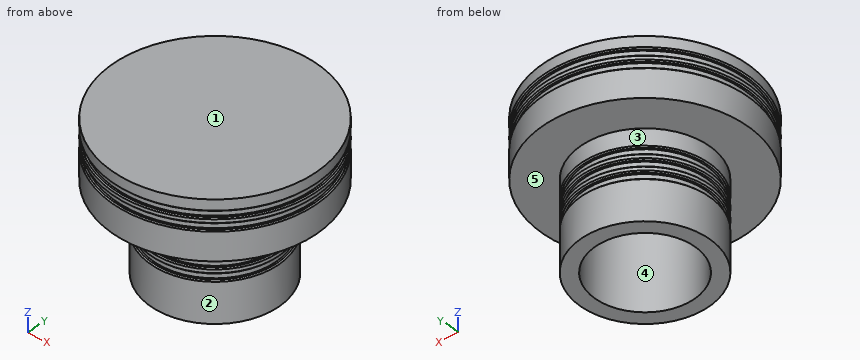
from build123d import *

# Parameters (mm, degrees)
F0_R      = 11
F0_R_2    = 8.5
F1_DEPTH  = 15
F2_R      = 17.5
F3_DEPTH  = 10
F4_R      = 11
F4_R_2    = 10.5
F5_DEPTH  = 12
F6_R      = 11
F6_R_2    = 10.5
F7_DEPTH  = 11
F8_R      = 11
F8_R_2    = 10.5
F9_DEPTH  = 10
F10_R     = 11
F10_R_2   = 10.5
F11_DEPTH = 9
F12_R     = 11
F12_R_2   = 10.5
F13_DEPTH = 8
F14_R     = 11
F14_R_2   = 10.5
F15_DEPTH = 7
F16_R     = 17.5
F16_R_2   = 17
F17_DEPTH = 8
F18_R     = 17.5
F18_R_2   = 17
F19_DEPTH = 7
F20_R     = 17.5
F20_R_2   = 17
F21_DEPTH = 6
F22_R     = 17.5
F22_R_2   = 17
F23_DEPTH = 5
F24_SIZE  = 0.2


with BuildPart() as f1:
    # F0 (on Top) → F1 (new body)
    with BuildSketch(Plane.XY):
        Circle(F0_R)
        Circle(F0_R_2, mode=Mode.SUBTRACT)
    extrude(amount=F1_DEPTH)

    # F2 (on face) → F3 (join)
    with BuildSketch(Plane.XY.offset(15)):
        Circle(F2_R)
    extrude(amount=F3_DEPTH)

    # F4 (on face) → F5 (cut)
    with BuildSketch(Plane(origin=(0, 0, 0), x_dir=(1, 0, 0), z_dir=(0, 0, -1))):
        Circle(F4_R)
        Circle(F4_R_2, mode=Mode.SUBTRACT)
    extrude(amount=-F5_DEPTH, mode=Mode.SUBTRACT)

    # F6 (on face) → F7 (join)
    with BuildSketch(Plane(origin=(0, 0, 0), x_dir=(1, 0, 0), z_dir=(0, 0, -1))):
        Circle(F6_R)
        Circle(F6_R_2, mode=Mode.SUBTRACT)
    extrude(amount=-F7_DEPTH)

    # F8 (on face) → F9 (cut)
    with BuildSketch(Plane(origin=(0, 0, 0), x_dir=(1, 0, 0), z_dir=(0, 0, -1))):
        Circle(F8_R)
        Circle(F8_R_2, mode=Mode.SUBTRACT)
    extrude(amount=-F9_DEPTH, mode=Mode.SUBTRACT)

    # F10 (on face) → F11 (join)
    with BuildSketch(Plane(origin=(0, 0, 0), x_dir=(1, 0, 0), z_dir=(0, 0, -1))):
        Circle(F10_R)
        Circle(F10_R_2, mode=Mode.SUBTRACT)
    extrude(amount=-F11_DEPTH)

    # F12 (on face) → F13 (cut)
    with BuildSketch(Plane(origin=(0, 0, 0), x_dir=(1, 0, 0), z_dir=(0, 0, -1))):
        Circle(F12_R)
        Circle(F12_R_2, mode=Mode.SUBTRACT)
    extrude(amount=-F13_DEPTH, mode=Mode.SUBTRACT)

    # F14 (on face) → F15 (join)
    with BuildSketch(Plane(origin=(0, 0, 0), x_dir=(1, 0, 0), z_dir=(0, 0, -1))):
        Circle(F14_R)
        Circle(F14_R_2, mode=Mode.SUBTRACT)
    extrude(amount=-F15_DEPTH)

    # F16 (on face) → F17 (cut)
    with BuildSketch(Plane(origin=(0, 0, 15), x_dir=(1, 0, 0), z_dir=(0, 0, -1))):
        Circle(F16_R)
        Circle(F16_R_2, mode=Mode.SUBTRACT)
    extrude(amount=-F17_DEPTH, mode=Mode.SUBTRACT)

    # F18 (on face) → F19 (join)
    with BuildSketch(Plane(origin=(0, 0, 15), x_dir=(1, 0, 0), z_dir=(0, 0, -1))):
        Circle(F18_R)
        Circle(F18_R_2, mode=Mode.SUBTRACT)
    extrude(amount=-F19_DEPTH)

    # F20 (on face) → F21 (cut)
    with BuildSketch(Plane(origin=(0, 0, 15), x_dir=(1, 0, 0), z_dir=(0, 0, -1))):
        Circle(F20_R)
        Circle(F20_R_2, mode=Mode.SUBTRACT)
    extrude(amount=-F21_DEPTH, mode=Mode.SUBTRACT)

    # F22 (on face) → F23 (join)
    with BuildSketch(Plane(origin=(0, 0, 15), x_dir=(1, 0, 0), z_dir=(0, 0, -1))):
        Circle(F22_R)
        Circle(F22_R_2, mode=Mode.SUBTRACT)
    extrude(amount=-F23_DEPTH)

    # F24
    f24_edges = [f1.edges().sort_by_distance(p)[0] for p in [
        (-17.5, 0, 23),
        (-17.5, 0, 22),
        (-17.5, 0, 20),
        (-17.5, 0, 21),
        (-11, 0, 12),
        (-11, 0, 10),
        (-11, 0, 11),
        (-11, 0, 9),
        (-11, 0, 8),
        (-11, 0, 7),
    ]]
    chamfer(f24_edges, length=F24_SIZE)


solid = f1.part
Read the model definition and answer for the solid it produces. Units are mm, in the model's axes. Face numbers are marked on the shaded views. A direction names the side the tool comes from. Give positions to 0.01 mm unless a question says otherwise; leave off trailing zeros. Write each loop counter-clockwise with the first axis right and the second up, starting at its lowest first coordinate (ties: lowest second). Pieces come first, ordered by that corner, then holes. Notation, with made-up numbers: (-39, 2.25) - (-31, 2.25) arc R17 ccw to (-31, 9.25) - close; hole circle Ø2 at (45, 77). An arc over 180 degrees is marked (long way). Use CSV: the item, a comma, the result in double quotes. Start each with the question number.
Item 1: Flat-ended cylindrical pins translate along their axes: P1, Ø8, axis at y = -12.5, z = 15, coming from the -X side; P2, Ø4, axis at y = 10.5, z = 13.5, coming from the -X side; P3, Ø2, axis at y = 2, z = 7.5, coming from the -X side. Find the tip coordinate at first contact, or state that the pin passes through.
Item 2: For the marked faces 1 and 2, determine the directions among +Z, -Z, +X, -X, +Y, -Y from which every point of the face is accessible in a straight line to the end or side of a thin tool.
Item 3: Consider line 1 (Z direction, x = 6.5, y = -8.5); line 2 (Y direction, x = 0, z = 10.25); line 3 (Z direction, x = -3.5, y = 0). Determine where each line is inside the solid, lowest interval first.
Item 4: The part is cut by section A-A, the plane z = 13.75. Give the vertices of the cut face in (x, y), and give its area (3 significant figures).
Item 5: The mould has two halves that part along X. Classify the marked faces 3, 4 and 5: pulls with the +X half, pulls with the -X half, needs draft (parallel to the pull), parting line crosses it, or undercut.
Taken from the geometry:
1,P1,"x = -15.3"
1,P2,"x = -14.9"
1,P3,"x = -10.92"
2,face 1,"+Z, +X, -X, +Y, -Y"
2,face 2,"-Z"
3,line 1,"0 to 7, 8 to 9, 10 to 11, 12 to 25"
3,line 2,"-11 to -8.5, 8.5 to 11"
3,line 3,"15 to 25"
4,outline,"circle Ø22 at (0, 0); hole circle Ø17 at (0, 0)"
4,area,"153 mm2"
5,face 3,"parting line crosses it"
5,face 4,"undercut"
5,face 5,"needs draft"
